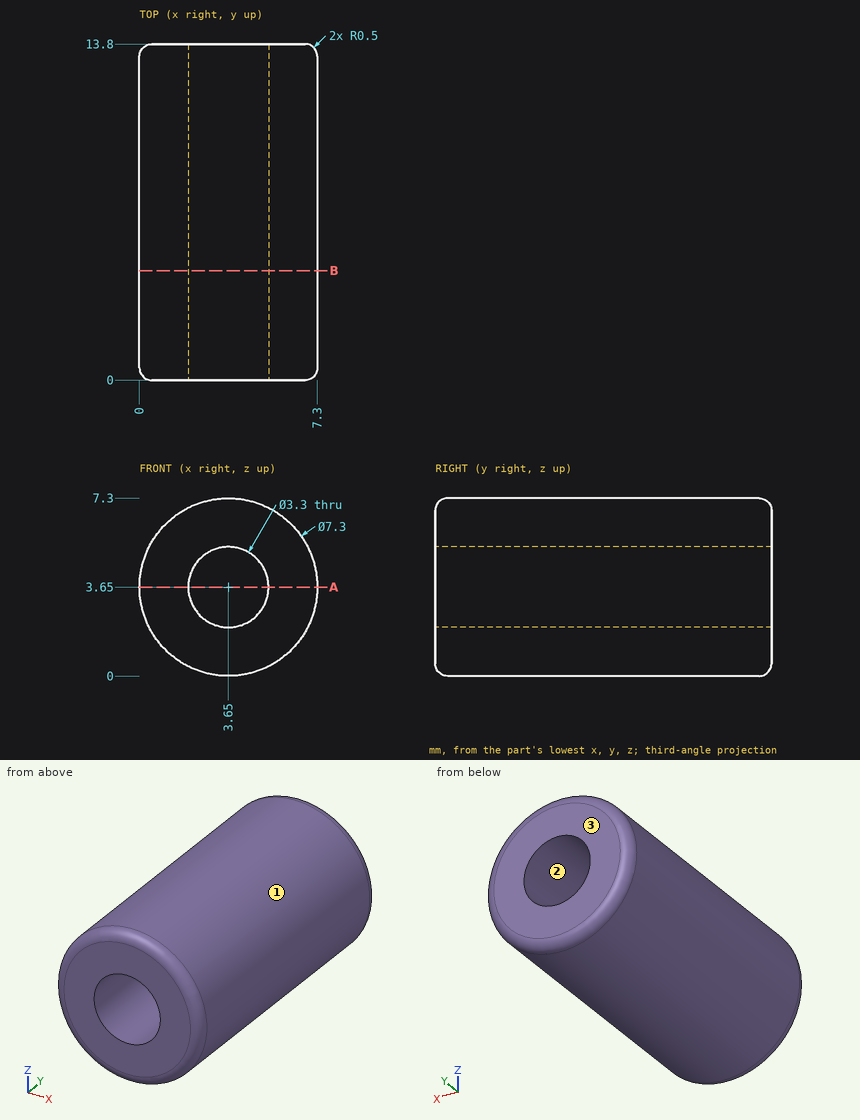
Part print with two shaded views. Sizes in mm from the minimum x, y, z corner. Round coordinates to 2 decimals unless told otherwise and drop trailing zeros. Order: outer loops, then holes, each group sorted by start corner. A loop starts at its lowest first (then second) coordinate and runs counter-clockwise, first axis right, second up.
(1) Band-saw the part on A-A (z = 3.65). List the corners of the cut face in (x, y).
(2) Pin check, flat tips, straight feed: pin 1 (2.5 mm diameter, centred on x = 3.65, z = 3.65, fed in from -Y); pin 2 (2 mm diameter, centred on y = 8, z = 1, fed in from +X); pin 3 (1.5 mm diameter, centred on x = 1.5, y = 8, fed in from -Z); pin 4 (3 mm diameter, centred on x = 3, y = 8, fed in from +Z). Stop position of each tip, or through.
(3) Drill centre lines: line 1 (X direction, y = 6.5, z = 5.5); line 2 (X direction, y = 1, z = 5); line 3 (Z direction, x = 3, y = 9.75). Where is each one in solid material? Low to high.
(4) Pull direction Z, two halves, no side cores. Call the marked faces 1, 2 and 3: released by +Z, released by -Z, zero draft, split by the parting line, or undercut.
(5) Band-saw the part on B-B (y = 4.5). List the corners of the cut face in (x, z), then the cut area to 3 significant figures.
Verdict:
1. outline: (0, 0.5) arc R0.5 ccw to (0.5, 0) - (2, 0) - (2, 13.8) - (0.5, 13.8) arc R0.5 ccw to (0, 13.3) - close; (5.3, 0) - (6.8, 0) arc R0.5 ccw to (7.3, 0.5) - (7.3, 13.3) arc R0.5 ccw to (6.8, 13.8) - (5.3, 13.8) - close
2. pin 1: passes through
2. pin 2: stops at x = 6.91
2. pin 3: stops at z = 0.28
2. pin 4: stops at z = 7.3
3. line 1: x = 0.5 to 6.8
3. line 2: x = 0.26 to 2.7, 4.6 to 7.04
3. line 3: z = 0.06 to 2.13, 5.17 to 7.24
4. face 1: split by the parting line
4. face 2: undercut
4. face 3: zero draft
5. outline: circle Ø7.3 at (3.65, 3.65); hole circle Ø3.3 at (3.65, 3.65)
5. area: 33.3 mm2
